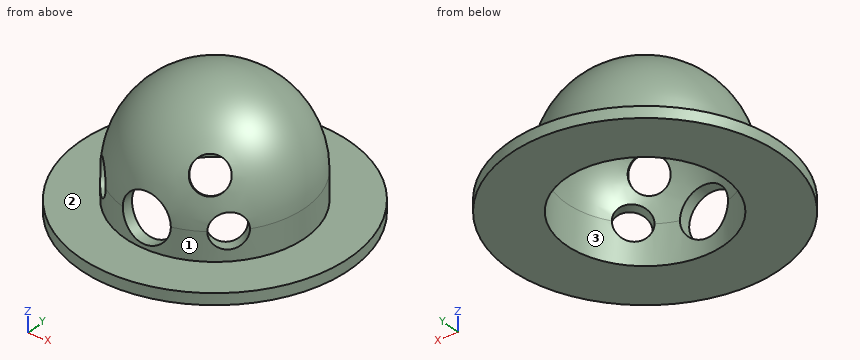
```python
from build123d import *

# Parameters (mm, degrees)
F2_R      = 4.25
F3_DEPTH  = 50
F6_R      = 3
F7_DEPTH  = 25
F13_R     = 3
F14_DEPTH = 25


with BuildPart() as f1:
    # F0 (on Front) → F1 (revolve)
    with BuildSketch(Plane.XZ):
        with BuildLine():
            Line((-24, -7), (-14, -7))
            Line((-14, -7), (-14, 0))
            ThreePointArc((-14, 0), (-9.8994949366, 9.8994949366), (0, 14))
            Line((0, 14), (0, 16))
            ThreePointArc((0, 16), (-11.313708499, 11.313708499), (-16, 0))
            Line((-16, 0), (-16, -5))
            Line((-16, -5), (-24, -5))
            Line((-24, -5), (-24, -7))
        make_face()
    revolve(axis=Axis((0, 0, 15), (0, 0, -1)))

    # F2 (on Front) → F3 (cut)
    with BuildSketch(Plane.XZ):
        Circle(F2_R)
    extrude(amount=F3_DEPTH, mode=Mode.SUBTRACT)

    # F6 (on face) → F7 (cut)
    with BuildSketch(Plane(origin=(0, 0, 0), x_dir=(-0.7071067812, 0.7071067812, 0), z_dir=(0.7071067812, 0.7071067812, 0))):
        Circle(F6_R)
    extrude(amount=-F7_DEPTH, mode=Mode.SUBTRACT)

    # F10 (on face) → F11 (revolve, cut)
    with BuildSketch(Plane(origin=(0, 0, 0), x_dir=(0, -1, 0), z_dir=(-0.7071067812, 0, 0.7071067812))):
        Polygon((3.9985278842, 3.9985278842), (16.6846810101, 16.6846810101), (14.5633606666, 18.8060013537), (1.8772075407, 6.1198482278), align=None)
    revolve(axis=Axis((7.3126186329, -10.3416044472, 7.3126186329), (0.5, -0.7071067812, 0.5)), mode=Mode.SUBTRACT)

    # F13 (on face) → F14 (cut)
    with BuildSketch(Plane(origin=(0, 0, 0), x_dir=(0.7071067812, 0.7071067812, 0), z_dir=(0.7071067812, -0.7071067812, 0))):
        Circle(F13_R)
    extrude(amount=F14_DEPTH, mode=Mode.SUBTRACT)


solid = f1.part
```
CAD build for the part. Positions are in the model's coordinates, mm. Face numbers are marked on the shaded views. Round coordinates to 2 decimals unless told otherwise and drop trailing zeros. Loops run counter-clockwise (first coordinate to the right, second up) from the corner with the lowest first, then second, coordinate; pieces in that order, holes last. Notation, with made-up numbers: M 13,78 L 40,78 A16 ccw 40,104 Z; hole C 85.5,45.25 d6. An arc over 180 degrees is marked long. Return JSON: item names as keys, results as strings. Group by question number.
(1) Mould opens along Y. For the marked faces 1, 2 and 3 say: +Y half, -Y half, draft (parallel to the pull), parting line (faces both ways), or undercut.
(2) Wall check: probe 1 along Z at (x, y) = (0, -14.1); probe 2 along Z at (x, y) = (13, -11); probe 3 along X at (y, z) = (4, 12). Give the ranges that are in metal, low to high. Write a range as [from, to].
(3) Drop flat-ended pins along their axis: P1, Ø10, axis at y = 8, z = 2.5, coming from the -X side; P2, Ø13.5, axis at x = 0, z = 0, coming from the +Y side; P3, Ø5, axis at x = -9, y = -1.5, coming from the +Z side. Give the stop position or say it passes through.
(4) Saw through at D-D, the plane y = -6. List the corners of the cut face in (x, z), and give its area (3 significant figures).
(5) Saw through at A-A, the plane x = 0. List the corners of the cut face in (y, z), and give its area (3 significant figures).
(6) Saw through at C-C, the plane z = 11.75. List the corners of the cut face in (x, y).
(7) Saw through at B-B, the plane y = 0. List the corners of the cut face in (x, z), and give its area (3 significant figures).
Answer list:
{
 "1": {"face 1": "parting line", "face 2": "draft", "face 3": "undercut"},
 "2": {"probe 1": "[-7, -4.25], [4.25, 7.56]", "probe 2": "[-7, -5]", "probe 3": "[-9.8, -6], [6, 9.8]"},
 "3": {"P1": "x = -15.64", "P2": "y = 24", "P3": "z = 14.56"},
 "4": {"outline": "M -23.24,-7 L -12.65,-7 L -12.65,0 A12.65 cw 12.65,0 L 12.65,-7 L 23.24,-7 L 23.24,-5 L 14.83,-5 L 14.83,0 A14.83 ccw -14.83,0 L -14.83,-5 L -23.24,-5 Z", "area": "158 mm2"},
 "5": {"outline": "M -24,-7 L -14,-7 L -14,-4.25 L -16,-4.25 L -16,-5 L -24,-5 Z; M -15.43,4.25 L -13.34,4.25 A14 cw 14,0 L 14,-7 L 24,-7 L 24,-5 L 16,-5 L 16,0 A16 ccw Z", "area": "137 mm2"},
 "6": {"outline": "C 0,0 d21.72; hole C 0,0 d15.22"},
 "7": {"outline": "M -24,-7 L -14,-7 L -14,0 A14 cw 14,0 L 14,-7 L 24,-7 L 24,-5 L 16,-5 L 16,0 A16 ccw -16,0 L -16,-5 L -24,-5 Z", "area": "154 mm2"}
}
